Answer from the drawing. Dimensions are ordinates in mm from the lowest x, y and z of the part. A direction names the side the tool comes from. Round coordinates to 2 decimals unless told otherwise and drop trailing zeros. Write each loop counter-clockwise with the first axis right and the second up, starting at its lowest first coordinate (ties: lowest second). Pieces come first, ordered by that corner, then holes. Notation, with made-up numbers: (2.5, 34) -> (39.5, 34) arc R15 ccw to (39.5, 48) -> close; hole circle Ø7 at (81.5, 64). An arc over 180 degrees is marked (long way). Return JSON: item names as keys, results as strings. Group by question number.
(1) A cutting plane is placed at C-C on z = 88.5. Give the vertices of the cut face in (x, y).
(2) For the marked faces 1 and 2, determine the directions among +Z, -Z, +X, -X, +Y, -Y from which every point of the face is accessible in a straight line to the end or side of a thin tool.
(3) Straight lines are drawn through the part: line 1 (X direction, y = 9, z = 70); line 2 (Y direction, x = 12, z = 1.65); line 3 (Z direction, x = 26, y = 1). For each, find the intervals that lie inside material, in ascending order.
(4) Given pin 1 (2.5 mm diameter, centred on x = 24, y = 5, fed in from +Z); pin 2 (4 mm diameter, centred on x = 13.5, y = 14, fed in from +Z), each flat-ended and moving along its own axis, determine where each tip first touches the part or whether it passes through.
(5) A cutting plane is placed at B-B on y = 5. Give the vertices of the cut face in (x, z), then the cut area to 3 significant figures.
(6) A cutting plane is placed at A-A on x = 24. Give the vertices of the cut face in (y, z), then the cut area to 3 significant figures.
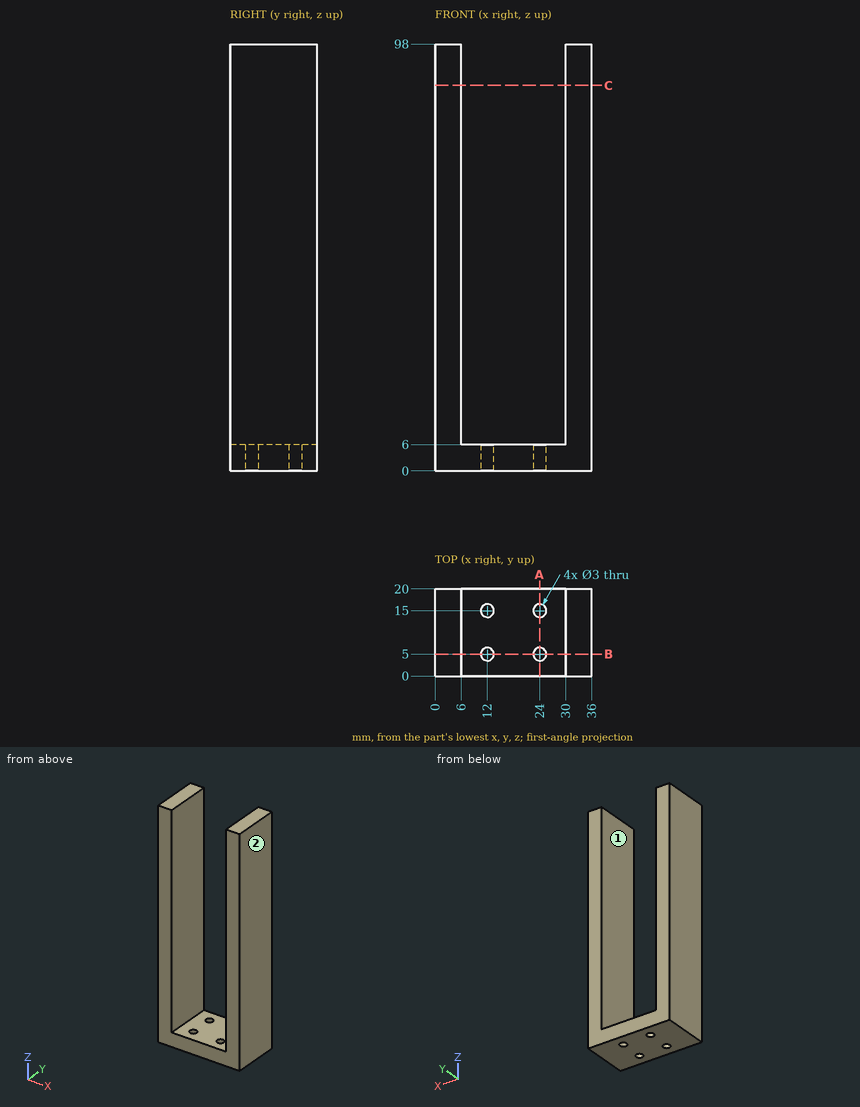
Checks:
{
 "1": {"outline": "(0, 0) -> (6, 0) -> (6, 20) -> (0, 20) -> close; (30, 0) -> (36, 0) -> (36, 20) -> (30, 20) -> close"},
 "2": {"face 1": "+Z, +Y, -Y", "face 2": "+Z, -Z, +X, +Y, -Y"},
 "3": {"line 1": "x = 0 to 6, 30 to 36", "line 2": "y = 0 to 3.5, 6.5 to 13.5, 16.5 to 20", "line 3": "z = 0 to 6"},
 "4": {"pin 1": "passes through", "pin 2": "stops at z = 6"},
 "5": {"outline": "(0, 0) -> (10.5, 0) -> (10.5, 6) -> (6, 6) -> (6, 98) -> (0, 98) -> close; (13.5, 0) -> (22.5, 0) -> (22.5, 6) -> (13.5, 6) -> close; (25.5, 0) -> (36, 0) -> (36, 98) -> (30, 98) -> (30, 6) -> (25.5, 6) -> close", "area": "1,280 mm^2"},
 "6": {"outline": "(0, 0) -> (3.5, 0) -> (3.5, 6) -> (0, 6) -> close; (6.5, 0) -> (13.5, 0) -> (13.5, 6) -> (6.5, 6) -> close; (16.5, 0) -> (20, 0) -> (20, 6) -> (16.5, 6) -> close", "area": "84.0 mm^2"}
}
